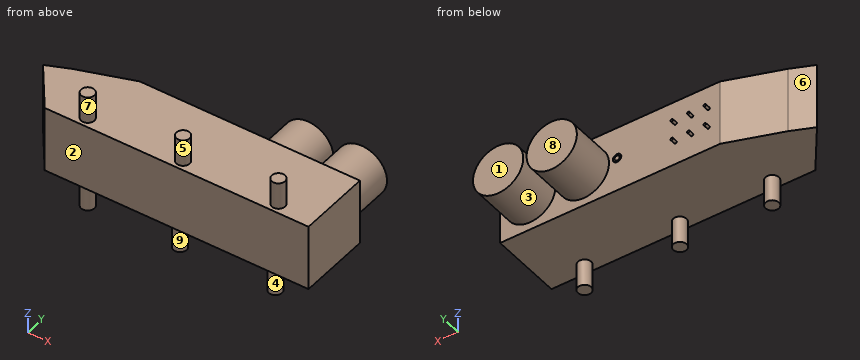
```python
from build123d import *

# Parameters (mm, degrees)
BOSS_EXTRUDE1_DEPTH     = 500
CUT_EXTRUDE2_DEPTH      = 1749.450897396
CUT_EXTRUDE2_DEPTH_BACK = 1749.450897396
SKETCH11_R              = 10
BOSS_EXTRUDE8_DEPTH     = 330
SKETCH12_R              = 50.165
BOSS_EXTRUDE14_DEPTH    = 203.2
BOSS_EXTRUDE15_START    = 203.2
SKETCH15_R              = 50.165
BOSS_EXTRUDE15_DEPTH    = 203.2
SKETCH17_R              = 50.292
BOSS_EXTRUDE16_DEPTH    = 203.2
SKETCH18_R              = 50.165
BOSS_EXTRUDE17_DEPTH    = 203.2
SKETCH9_R               = 190.5
BOSS_EXTRUDE19_DEPTH    = 635
SKETCH19_R              = 31.75
SKETCH19_R_2            = 19.05
CUT_EXTRUDE5_DEPTH      = 25.4


with BuildPart() as part:
    # Sketch2 → Boss-Extrude1 (new body)
    with BuildSketch(Plane.XY):
        Polygon((-600, 76.079136691), (-100, 290.827338129), (1650, 290.827338129), (1650, -259.172661871), (-350, -259.172661871), align=None)
    extrude(amount=BOSS_EXTRUDE1_DEPTH)

    # Sketch3 → Cut-Extrude2 (cut, two sides: drawn at the far end of the back side and taken through both)
    with BuildSketch(Plane.XY.offset(-CUT_EXTRUDE2_DEPTH_BACK)):
        Polygon((-629.160159728, 80.318281341), (0, 297.197748554), (-133.945595933, 297.197748554), align=None)
    extrude(amount=CUT_EXTRUDE2_DEPTH + CUT_EXTRUDE2_DEPTH_BACK, mode=Mode.SUBTRACT)

    # Sketch11 → Boss-Extrude8 (add)
    with BuildSketch(Plane(origin=(0, 0, 0), x_dir=(1, 0, 0), z_dir=(0, 1, 0))):
        with Locations((320.593573559, -323.788946962)):
            Circle(SKETCH11_R)
        with Locations(Location((70.593573559, -323.788946962, 0), (0, 0, 90))):
            Circle(SKETCH11_R)
        with Locations((195.593573559, -322.326233751)):
            Circle(SKETCH11_R)
        with Locations(Location((320.593573559, -173.125553361, 0), (0, 0, 90))):
            Circle(SKETCH11_R)
        with Locations(Location((195.593573559, -173.125553361, 0), (0, 0, 90))):
            Circle(SKETCH11_R)
        with Locations((70.593573559, -173.125553361)):
            Circle(SKETCH11_R)
    extrude(amount=BOSS_EXTRUDE8_DEPTH)

    # Sketch12 → Boss-Extrude14 (add)
    with BuildSketch(Plane(origin=(0, 0, 0), x_dir=(-1, 0, 0), z_dir=(0, 0, -1))):
        with Locations(Location((-1345.2, -182.972661871, 0), (0, 0, 180))):
            Circle(SKETCH12_R)
        with Locations(Location((77.2, -182.972661871, 0), (0, 0, 180))):
            Circle(SKETCH12_R)
    extrude(amount=BOSS_EXTRUDE14_DEPTH)

    # Sketch15 → Boss-Extrude15 (add)
    with BuildSketch(Plane.XY.offset(500).offset(BOSS_EXTRUDE15_START)):
        with Locations((1368.06, -182.972661871)):
            Circle(SKETCH15_R)
        with Locations((-77.2, -182.972661871)):
            Circle(SKETCH15_R)
    extrude(amount=-BOSS_EXTRUDE15_DEPTH)

    # Sketch17 → Boss-Extrude16 (add, through all)
    with BuildSketch(Plane.XY.offset(500)):
        with Locations((645.43, -182.972661871)):
            Circle(SKETCH17_R)
    extrude(amount=BOSS_EXTRUDE16_DEPTH)

    # Sketch18 → Boss-Extrude17 (add, through all)
    with BuildSketch(Plane(origin=(0, 0, 0), x_dir=(-1, 0, 0), z_dir=(0, 0, -1))):
        with Locations(Location((-622.57, -182.972661871, 0), (0, 0, 180))):
            Circle(SKETCH18_R)
    extrude(amount=BOSS_EXTRUDE17_DEPTH)

    # Sketch9 → Boss-Extrude19 (add)
    with BuildSketch(Plane(origin=(0, 0, 0), x_dir=(1, 0, 0), z_dir=(0, 1, 0))):
        with Locations(Location((1421.4, -248.149283127, 0), (0, 0, 90))):
            Circle(SKETCH9_R)
        with Locations(Location((1015, -248.149283127, 0), (0, 0, 90))):
            Circle(SKETCH9_R)
    extrude(amount=BOSS_EXTRUDE19_DEPTH)

    # Sketch19 → Cut-Extrude5 (cut)
    with BuildSketch(Plane(origin=(0, 290.827338129, 0), x_dir=(1, 0, 0), z_dir=(0, 1, 0))):
        with Locations(Location((763.220602861, -258.539612091, 0), (0, 0, 180))):
            Circle(SKETCH19_R)
        with Locations(Location((763.220602861, -258.539612091, 0), (0, 0, 180))):
            Circle(SKETCH19_R_2, mode=Mode.SUBTRACT)
    extrude(amount=-CUT_EXTRUDE5_DEPTH, mode=Mode.SUBTRACT)


solid = part.part
```
The listing builds one solid part. Answer for the finished solid, in the listing's coordinates (mm). Face numbers are marked on the shaded views. A direction names the side the tool comes from. Give positions to 0.01 mm unless a question says otherwise; leave off trailing zeros. Order: outer loops, then holes, each group sorted by start corner. A loop starts at its lowest first (then second) coordinate and runs counter-clockwise, first axis right, second up. Notation, with made-up numbers: (83.25, 59) -> (131.25, 59) arc R14 cw to (131.25, 64) -> close; hole circle Ø10 at (62.5, 3). An arc over 180 degrees is marked (long way). One line per item, written item: value.
1) Find section A-A, the plane x = 1015. Determine the outline of the cut face in (y, z).
Reported:
outline: (-259.17, 0) -> (290.83, 0) -> (290.83, 57.65) -> (635, 57.65) -> (635, 438.65) -> (290.83, 438.65) -> (290.83, 500) -> (-259.17, 500) -> close
2) Find the intervals of material crossed by line 1 (Y direction, x = 608, z = 373); line 2 (Z direction, x = 257.5, y = 204.5); line 3 (X direction, y = 502.5, z = 98.5), in increasing order.
Reported:
line 1: y = -259.17 to 290.83
line 2: z = 0 to 500
line 3: x = 897.12 to 1132.88, 1303.52 to 1539.28
3) Flat-ended cylindrical pins translate along their axes: P1, Ø1.5, axis at y = -53, z = 212.5, coming from the -X side; P2, Ø6, axis at x = 325.5, z = 170.5, coming from the +Y side; P3, Ø4, axis at x = 1142.5, y = 381, coming from the +Z side. Find the tip coordinate at first contact, or state that the pin passes through.
Reported:
P1: stops at x = -504.3
P2: stops at y = 330
P3: stops at z = 391.47
4) Find section B-B, the plane z = 124. Determine the outline of the cut face in (x, y), plus the area to 3 significant figures.
Reported:
outline: (-600, 76.08) -> (-350, -259.17) -> (1650, -259.17) -> (1650, 290.83) -> (1565.89, 290.83) -> (1565.89, 635) -> (1276.91, 635) -> (1276.91, 290.83) -> (1159.49, 290.83) -> (1159.49, 635) -> (870.51, 635) -> (870.51, 290.83) -> (-18.48, 290.83) -> (-431.44, 148.47) -> close
area: 1,340,000 mm^2
5) Find section D-D, the plane z = 592. Determine the outline of the cut face in (x, y) (3 decimals), plus the area to 3 significant figures.
Reported:
outline: circle Ø100.33 at (-77.2, -182.973); circle Ø100.584 at (645.43, -182.973); circle Ø100.33 at (1368.06, -182.973)
area: 23,800 mm^2
6) A tool of negligible diameter and unlimited length cuts with its end or side. For the marked faces 1, 2, 3, 4 and 5, from which of +Z, -Z, +X, -X, +Y, -Y can it reach the whole face along a straight path? Write none if from no direction.
Reported:
face 1: +Z, -Z, +X, -X, +Y
face 2: +Z, -Z, +X, -X, -Y
face 3: +Y
face 4: -Z
face 5: +Z
7) Determine the mould class of the marked faces 6, 7, 8 and 9 for opening direction X: pulls with the +X half, pulls with the -X half, needs draft (parallel to the pull), parting line crosses it, or undercut.
Reported:
face 6: pulls with the -X half
face 7: undercut
face 8: needs draft
face 9: undercut
8) Find section C-C, the plane y = 454.5. Determine the outline of the cut face in (x, z).
Reported:
outline: circle Ø381 at (1015, 248.15); circle Ø381 at (1421.4, 248.15)
